from build123d import *

# Parameters (mm, degrees)
SKETCH1_W           = 75
SKETCH1_H           = 75
BOSS_EXTRUDE1_DEPTH = 75
SKETCH2_R           = 12.5
CUT_EXTRUDE1_DEPTH  = 92.855865354
SKETCH5_R           = 12.5
CUT_EXTRUDE2_DEPTH  = 113.5


with BuildPart() as part:
    # Sketch1 → Boss-Extrude1 (new body)
    with BuildSketch(Plane(origin=(0, 0, 0), x_dir=(1, 0, 0), z_dir=(0, 1, 0))):
        Rectangle(SKETCH1_W, SKETCH1_H)
    extrude(amount=BOSS_EXTRUDE1_DEPTH)

    # Sketch2 → Cut-Extrude1 (cut, through all)
    with BuildSketch(Plane(origin=(0, 0, 0), x_dir=(-1, 0, 0), z_dir=(0, -1, 0))):
        with Locations(Location((0, 0, 0), (0, 0, 90))):
            Circle(SKETCH2_R)
    extrude(amount=-CUT_EXTRUDE1_DEPTH, mode=Mode.SUBTRACT)

    # Sketch5 → Cut-Extrude2 (cut, through all)
    with BuildSketch(Plane(origin=(37.5, 0, 0), x_dir=(0, 0, -1), z_dir=(1, 0, 0))):
        with Locations((0, 37.5)):
            Circle(SKETCH5_R)
    extrude(amount=-CUT_EXTRUDE2_DEPTH, mode=Mode.SUBTRACT)


solid = part.part
Geometry: final body of the model. Coordinates: model frame, mm. Coordinates: 2 decimals unless noted, no trailing zeros. Loops run counter-clockwise (first coordinate to the right, second up) from the corner with the lowest first, then second, coordinate; pieces in that order, holes last. Notation, with made-up numbers: (6.5, 58) - (14.5, 58) arc R16 ccw to (14.5, 68) - close; hole circle Ø3 at (-31.75, -16). An arc over 180 degrees is marked (long way). Put each result on its own line as item: value. Start each with the question number.
Q1. Line query: line 1 (X direction, y = 67.5, z = 0); line 2 (Z direction, x = 24, y = 37); line 3 (Y direction, x = 14.5, z = 0). Output: solid intervals per line, ascending.
Q2. Cut plane D-D, the plane y = 9.5. Return loops of the section in (x, z).
Q3. Cut plane C-C, the plane x = -11. Return loops of the section in (y, z).
Q4. Pull-direction query (X, two-part tool) for faces 1 (the flat face through (-1, 37, -37.5)), 2 (the cylindrical face through (0.55, 60.154, 12.488)), 3 (the flat face through (-37.5, 37, 17)); classes: released by +X, released by -X, zero draft, split by the parting line, or undercut.
Q5. Cut plane B-B, the plane z = 0. Return loops of the section in (x, y), and give its area (3 significant figures).
Q6. Pin query (flat end, axial travel): pin 1 Ø22.5 at (y, z) = (37.5, 0) entering from +X. Return the tip coordinate at first contact, or that it passes through.
Q7. Cut plane A-A, the plane y = 34. Return loops of the section in (x, z).
Filled sheet:
1. line 1: -37.5 to -12.5, 12.5 to 37.5
1. line 2: -37.5 to -12.49, 12.49 to 37.5
1. line 3: 0 to 25, 50 to 75
2. outline: (-37.5, -37.5) - (37.5, -37.5) - (37.5, 37.5) - (-37.5, 37.5) - close; hole circle Ø25 at (0, 0)
3. outline: (0, -37.5) - (75, -37.5) - (75, -5.94) - (48.5, -5.94) arc R12.5 cw to (26.5, -5.94) - (0, -5.94) - close; (0, 5.94) - (26.5, 5.94) arc R12.5 cw to (48.5, 5.94) - (75, 5.94) - (75, 37.5) - (0, 37.5) - close
4. face 1: zero draft
4. face 2: undercut
4. face 3: released by -X
5. outline: (-37.5, 0) - (-12.5, 0) - (-12.5, 25) - (-37.5, 25) - close; (-37.5, 50) - (-12.5, 50) - (-12.5, 75) - (-37.5, 75) - close; (12.5, 0) - (37.5, 0) - (37.5, 25) - (12.5, 25) - close; (12.5, 50) - (37.5, 50) - (37.5, 75) - (12.5, 75) - close
5. area: 2,500 mm²
6. pin 1: through
7. outline: (-37.5, -37.5) - (37.5, -37.5) - (37.5, -12) - (3.5, -12) arc R12.5 cw to (-3.5, -12) - (-37.5, -12) - close; (-37.5, 12) - (-3.5, 12) arc R12.5 cw to (3.5, 12) - (37.5, 12) - (37.5, 37.5) - (-37.5, 37.5) - close
